```python
from build123d import *

# Parameters (mm, degrees)
CROQUIS1_W              = 91.2
CROQUIS1_H              = 54
SALIENTE_EXTRUIR1_DEPTH = 2
CROQUIS2_W              = 91.2
CROQUIS2_H              = 54
CROQUIS2_W_2            = 89.2
CROQUIS2_H_2            = 52
SALIENTE_EXTRUIR2_DEPTH = 3
CROQUIS3_W              = 87.2
CROQUIS3_H              = 50
CROQUIS3_W_2            = 81.2
CROQUIS3_H_2            = 44
SALIENTE_EXTRUIR3_DEPTH = 9
REDONDEO1_SIZE          = 3
CROQUIS4_W              = 32
CROQUIS4_H              = 8
CORTAR_EXTRUIR2_DEPTH   = 28
CROQUIS5_R              = 10.16
CROQUIS5_W              = 5
CROQUIS5_H              = 5
CORTAR_EXTRUIR3_DEPTH   = 28
CROQUIS6_W              = 12
CROQUIS6_H              = 6
CORTAR_EXTRUIR4_DEPTH   = 7


with BuildPart() as part:
    # Croquis1 → Saliente-Extruir1 (new body)
    with BuildSketch(Plane(origin=(0, 0, 0), x_dir=(1, 0, 0), z_dir=(0, 1, 0))):
        Rectangle(CROQUIS1_W, CROQUIS1_H)
    extrude(amount=SALIENTE_EXTRUIR1_DEPTH)

    # Croquis2 → Saliente-Extruir2 (add)
    with BuildSketch(Plane(origin=(0, 2, 0), x_dir=(1, 0, 0), z_dir=(0, 1, 0))):
        Rectangle(CROQUIS2_W, CROQUIS2_H)
        Rectangle(CROQUIS2_W_2, CROQUIS2_H_2, mode=Mode.SUBTRACT)
    extrude(amount=SALIENTE_EXTRUIR2_DEPTH)

    # Croquis3 → Saliente-Extruir3 (add)
    with BuildSketch(Plane(origin=(0, 2, 0), x_dir=(1, 0, 0), z_dir=(0, 1, 0))):
        Rectangle(CROQUIS3_W, CROQUIS3_H)
        Rectangle(CROQUIS3_W_2, CROQUIS3_H_2, mode=Mode.SUBTRACT)
    extrude(amount=SALIENTE_EXTRUIR3_DEPTH)

    # Redondeo1
    # a fillet whose section is not a circle: 3 mm, written as the material it takes off along each edge
    with BuildSketch(Plane(origin=(51.1, 11, -25), x_dir=(0, -1, 0), z_dir=(-1, 0, 0)), Plane(origin=(-51.1, 11, 25), x_dir=(0, -1, 0), z_dir=(1, 0, 0))) as redondeo1_piece_1:
        with BuildLine():
            Bezier((REDONDEO1_SIZE, 0), (0, 0), (0, REDONDEO1_SIZE), weights=[1, 0.111111111, 1])
            Line((0, REDONDEO1_SIZE), (0, 0))
            Line((0, 0), (REDONDEO1_SIZE, 0))
        make_face()
    extrude(amount=102.2, mode=Mode.SUBTRACT)
    with BuildSketch(Plane(origin=(43.6, 11, 32.5), x_dir=(0, -1, 0), z_dir=(0, 0, -1)), Plane(origin=(-43.6, 11, -32.5), x_dir=(0, -1, 0), z_dir=(0, 0, 1))) as redondeo1_piece_2:
        with BuildLine():
            Bezier((REDONDEO1_SIZE, 0), (0, 0), (0, REDONDEO1_SIZE), weights=[1, 0.111111111, 1])
            Line((0, REDONDEO1_SIZE), (0, 0))
            Line((0, 0), (REDONDEO1_SIZE, 0))
        make_face()
    extrude(amount=65, mode=Mode.SUBTRACT)

    # Croquis4 → Cortar-Extruir2 (cut)
    with BuildSketch(Plane(origin=(0, 2, 0), x_dir=(1, 0, 0), z_dir=(0, 1, 0))):
        with Locations((-27.6, 21)):
            Rectangle(CROQUIS4_W, CROQUIS4_H)
    extrude(amount=CORTAR_EXTRUIR2_DEPTH, mode=Mode.SUBTRACT)

    # Croquis5 → Cortar-Extruir3 (cut)
    with BuildSketch(Plane.XZ):
        with Locations(Location((26.4, 1.8, 0), (0, 0, 270))):
            Circle(CROQUIS5_R)
        with Locations((1.1, 12.5)):
            Rectangle(CROQUIS5_W, CROQUIS5_H)
        with Locations((1.1, -12.5)):
            Rectangle(CROQUIS5_W, CROQUIS5_H)
    extrude(amount=-CORTAR_EXTRUIR3_DEPTH, mode=Mode.SUBTRACT)

    # Croquis6 → Cortar-Extruir4 (cut)
    with BuildSketch(Plane(origin=(0, 0, -27), x_dir=(-1, 0, 0), z_dir=(0, 0, -1))):
        with Locations((28, 5)):
            Rectangle(CROQUIS6_W, CROQUIS6_H)
    extrude(amount=-CORTAR_EXTRUIR4_DEPTH, mode=Mode.SUBTRACT)


solid = part.part
```
Verification items for the finished model (mm, model axes). A direction names the side the tool comes from. Coordinates: 2 decimals unless noted, no trailing zeros. Return JSON: item names as keys, results as strings.
(1) Go/stop test with flat-tipped pins: pin 1 (12 mm diameter, centred on x = -8.5, z = 17, fed in from +Y); pin 2 (5 mm diameter, centred on y = 9, z = 20.5, fed in from +X); pin 3 (1.5 mm diameter, centred on x = -29, y = 3.5, fed in from -Z); pin 4 (1 mm diameter, centred on y = 8.5, z = 17, fed in from -X). Record where each tip stops, or that it passes through.
Filled sheet:
{"pin 1": "stops at y = 11", "pin 2": "stops at x = 43.6", "pin 3": "stops at z = 22", "pin 4": "stops at x = -43.6"}
(2) Mould release check, pull along X, two halves, no side actions. Record for faces 1 (the flat face through (-1, 2, 27)), 2 (the flat face through (16, 5, -25)), 3 (the flat face through (-45.6, 2, 0)): pulls with the +X half, pulls with the -X half, needs draft (parallel to the pull), parting line crosses it, or undercut.
Filled sheet:
{"face 1": "needs draft", "face 2": "undercut", "face 3": "pulls with the -X half"}
(3) Access from +Z, -Z, +X, -X, +Y, -Y to the whole of each face (thin tool, end or side, straight path). Record for faces 4 (the flat face through (40.6, 6, 0)), 5 (the flat face through (-1, 2, -27)), 6 (the flat face through (-1.4, 1, 12)).
Filled sheet:
{"face 4": "+Y", "face 5": "-Z, +X, -X, +Y, -Y", "face 6": "+Y, -Y"}
(4) Thickness scan on line 1 along X through (y, z) = (4.5, 15.5); line 2 along Z through (x, y) = (34, 4); line 3 along Z through (x, y) = (-12, 3). Record the ranges inside material, lowest first.
Filled sheet:
{"line 1": "x = -45.6 to -44.6, -43.6 to -40.6, 40.6 to 43.6, 44.6 to 45.6", "line 2": "z = -27 to -26, -25 to -22, 22 to 25, 26 to 27", "line 3": "z = -27 to -26, 22 to 25, 26 to 27"}
